CAD build for the part. Positions are in the model's coordinates, mm. Coordinates: 2 decimals unless noted, no trailing zeros. Loops run counter-clockwise (first coordinate to the right, second up) from the corner with the lowest first, then second, coordinate; pieces in that order, holes last. Notation, with made-up numbers: (85.5, 5) - (104.5, 5) arc R18 cw to (104.5, 29) - close; hole circle Ø1 at (69.25, 22). An arc over 180 degrees is marked (long way). Put each result on its own line as item: value.
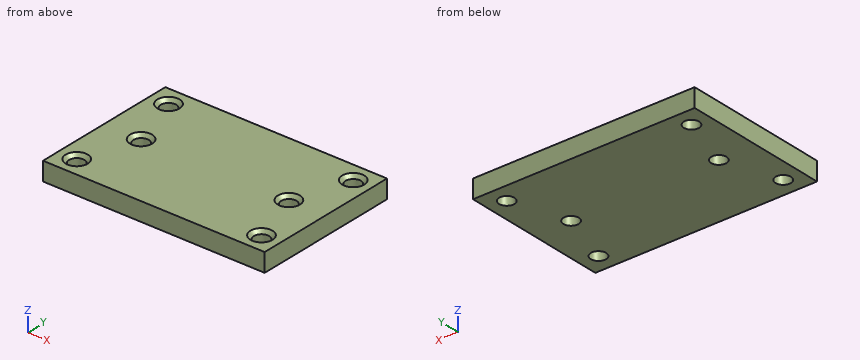
Autodesk Inventor part; units mm, degrees
ref_plane "YZ Plane" through (0, 0, 0) normal (1, 0, 0) x (0, 1, 0)
ref_plane "XZ Plane" through (0, 0, 0) normal (0, 1, 0) x (-1, 0, 0)
ref_plane "XY Plane" through (0, 0, 0) normal (0, 0, 1) x (1, 0, 0)
sketch "Szkic1" plane through (0, 0, 0) normal (0, 0, 1) x (1, 0, 0)
  line L0 (21.4781, -20) -> (21.4781, 20)
  line L1 (-21.5797, -20) -> (21.4781, -20)
  line L2 (-38.5219, 20) -> (-38.5219, -20)
  line L3 (-38.5219, -20) -> (-25.4723, -20)
  line L4 (-25.4723, -20) -> (-21.5797, -20)
  line L5 (-31.9971, 20) -> (-38.5219, 20)
  line L6 (21.4781, 20) -> (6.0004, 20)
  line L7 (6.0004, 20) -> (-31.9971, 20)
  point P0 (0, 0)
extrude "Wyciągnięcie proste1" add sketch "Szkic1" along normal blind 5
sketch "Szkic2" plane through (0, 0, 5) normal (0, 0, 1) x (1, 0, 0)
  circle A0 centre (16.4781, 15) radius 2.067
  circle A1 centre (16.4781, -15) radius 2.067
  circle A2 centre (-33.5219, -15) radius 2.067
  circle A3 centre (-33.5219, 15) radius 2.067
  point P0 (0, 0)
hole "Otwór1" at (16.4781, -15, 5) at (-33.5219, -15, 5) at (16.4781, 15, 5) at (-33.5219, 15, 5) direction (0, 0, -1) diameter 4.134 end through all countersink diameter 6 countersink angle 90
sketch "Szkic3" plane through (0, 0, 5) normal (0, 0, 1) x (1, 0, 0)
  line L0 (21.4781, 20) -> (-38.5219, 20)
  line L1 (21.4781, -20) -> (21.4781, 20)
  line L2 (-38.5219, 20) -> (-38.5219, -20)
  point P0 (0, 0)
  point P1 (11.4781, 0)
  point P2 (-28.5219, 0)
  dimension "d9" = 20
  dimension "d10" = 10
  dimension "d11" = 20
  dimension "d12" = 10
hole "Otwór2" at (11.4781, 0, 5) at (-28.5219, 0, 5) direction (0, 0, -1) diameter 4.134 end through all countersink diameter 6 countersink angle 90
properties part number "podstawka"
Q1. Slice it at B-B, the plane z = 1.65. Give the cut face in (x, y), then the cut area to 3 significant figures.
Determined:
outline: (-38.52, -20) - (21.48, -20) - (21.48, 20) - (-38.52, 20) - close; hole circle Ø4.13 at (-33.52, -15); hole circle Ø4.13 at (-33.52, 15); hole circle Ø4.13 at (-28.52, 0); hole circle Ø4.13 at (11.48, 0); hole circle Ø4.13 at (16.48, -15); hole circle Ø4.13 at (16.48, 15)
area: 2,320 mm2
Q2. Wall check: L1, parallel to X at y = 0, z = 3.25; L2, parallel to X at y = -15, z = 1.5; L3, parallel to Y at x = -32, z = 4.85. Give the ranges that are in metal, low to high. Write a range as from..to.
Determined:
L1: -38.52..-30.59, -26.45..9.41, 13.55..21.48
L2: -38.52..-35.59, -31.45..14.41, 18.55..21.48
L3: -20..-17.41, -12.59..12.59, 17.41..20
Q3. Slice it at A-A, the plane y = 15. Give the cut face in (x, z), then the cut area to 3 significant figures.
Determined:
outline: (-38.52, 0) - (-35.59, 0) - (-35.59, 4.07) - (-36.52, 5) - (-38.52, 5) - close; (-31.45, 0) - (14.41, 0) - (14.41, 4.07) - (13.48, 5) - (-30.52, 5) - (-31.45, 4.07) - close; (18.55, 0) - (21.48, 0) - (21.48, 5) - (19.48, 5) - (18.55, 4.07) - close
area: 257 mm2
Q4. Pin check, flat tip, straight feed: pin 1 Ø3.5 at (x, y) = (16.48, -15) entering from +Z. Stop position of the tip, or through.
Determined:
pin 1: through
